Build history of the part. All positions in model axes, mm. A direction names the side the tool comes from. Give positions to 0.01 mm unless a question says otherwise; leave off trailing zeros. Order: outer loops, then holes, each group sorted by start corner. A loop starts at its lowest first (then second) coordinate and runs counter-clockwise, first axis right, second up. Notation, with made-up numbers: (2.25, -16.5) - (27.25, -16.5) arc R17 cw to (27.25, 4.5) - close; hole circle Ø1 at (54, 55). An arc over 180 degrees is marked (long way). Write each question's results on one line, items separated by ' | '. Start each with the question number.
from build123d import *

# Parameters (mm, degrees)
SKETCH1_W             = 80
SKETCH1_H             = 100
BOSS_EXTRUDE1_DEPTH   = 3.5
SKETCH3_W             = 56
SKETCH3_H             = 88
BOSS_EXTRUDE2_DEPTH   = 21.5
SKETCH4_W             = 50
SKETCH4_H             = 82
CUT_EXTRUDE4_DEPTH    = 16
CUT_EXTRUDE5_DEPTH    = 6
SKETCH8_W             = 30
SKETCH8_H             = 5
CUT_EXTRUDE6_DEPTH    = 6
CUT_EXTRUDE7_REACH    = 112.567
SKETCH9_W             = 40
SKETCH9_H             = 12
F_4_0MM_DOWEL_HOLE1_D = 4
FILLET1_R             = 7
FILLET2_R             = 2
FILLET3_R             = 1
FILLET4_R             = 2


# Some blends are built 0.0001 mm under size
with BuildPart() as part:
    # Sketch1 → Boss-Extrude1 (new body)
    with BuildSketch(Plane.XY):
        Rectangle(SKETCH1_W, SKETCH1_H)
    extrude(amount=BOSS_EXTRUDE1_DEPTH)

    # Sketch3 → Boss-Extrude2 (add)
    with BuildSketch(Plane.XY.offset(3.5)):
        Rectangle(SKETCH3_W, SKETCH3_H)
    extrude(amount=BOSS_EXTRUDE2_DEPTH)

    # Sketch4 → Cut-Extrude4 (cut)
    with BuildSketch(Plane(origin=(0, 0, 0), x_dir=(-1, 0, 0), z_dir=(0, 0, -1))):
        Rectangle(SKETCH4_W, SKETCH4_H)
    extrude(amount=-CUT_EXTRUDE4_DEPTH, mode=Mode.SUBTRACT)

    # Sketch7 → Cut-Extrude5 (cut)
    with BuildSketch(Plane(origin=(0, 0, 16), x_dir=(-1, 0, 0), z_dir=(0, 0, -1))):
        Polygon((-18, 41), (18, 41), (18, 34), (25, 34), (25, -34), (18, -34), (18, -41), (-18, -41), (-18, -34), (-25, -34), (-25, 34), (-18, 34), align=None)
    extrude(amount=-CUT_EXTRUDE5_DEPTH, mode=Mode.SUBTRACT)

    # Sketch8 → Cut-Extrude6 (cut)
    with BuildSketch(Plane.XY.offset(25)):
        with Locations((0, -17)):
            Rectangle(SKETCH8_W, SKETCH8_H)
    cut_extrude6 = extrude(amount=-CUT_EXTRUDE6_DEPTH, mode=Mode.SUBTRACT)

    # Mirror1: Cut-Extrude6 across plane
    add(cut_extrude6.mirror(Plane.ZX), mode=Mode.SUBTRACT)

    # Sketch9 → Cut-Extrude7 (cut, up to next)
    with BuildSketch(Plane.XZ.offset(50), mode=Mode.PRIVATE) as cut_extrude7_sk1:
        with Locations((0, 6)):
            Rectangle(SKETCH9_W, SKETCH9_H)
    cut_extrude7_tool1 = extrude(cut_extrude7_sk1.sketch, amount=-CUT_EXTRUDE7_REACH, mode=Mode.PRIVATE) & part.part
    add(cut_extrude7_tool1.solids().sort_by_distance((0, -50, 6))[0], mode=Mode.SUBTRACT)

    # Ø4.0mm Dowel Hole1 (through all)
    with Locations(Plane(origin=(0, 0, 0), x_dir=(-1, 0, 0), z_dir=(0, 0, -1))):
        with Locations((-35, 45), (35, 45), (35, -45), (-35, -45)):
            Hole(F_4_0MM_DOWEL_HOLE1_D / 2)

    # Fillet1
    fillet1_edges = [part.edges().sort_by_distance(p)[0] for p in [
        (-18, 34, 19),
        (18, 34, 19),
        (18, -34, 19),
        (-18, -34, 19),
    ]]
    fillet(fillet1_edges, radius=FILLET1_R - 0.0001)  # a hair under: the kernel refuses the full size

    # Fillet2
    fillet2_edges = [part.edges().sort_by_distance(p)[0] for p in [
        (28, -44, 14.25),
        (28, 44, 14.25),
        (-28, 44, 14.25),
        (-28, -44, 14.25),
        (28, 0, 25),
        (0, 44, 25),
        (-28, 0, 25),
        (15, -14.5, 23.5),
        (15, -19.5, 23.5),
        (-15, -19.5, 23.5),
        (-15, -14.5, 23.5),
        (15, 19.5, 23.5),
        (15, 14.5, 23.5),
        (-15, 14.5, 23.5),
        (-15, 19.5, 23.5),
    ]]
    fillet(fillet2_edges, radius=FILLET2_R)

    # Fillet3
    fillet3_edges = [part.edges().sort_by_distance(p)[0] for p in [
        (-40, 0, 3.5),
        (23, -44, 3.5),
        (30, -50, 3.5),
        (-30, -50, 3.5),
        (28, 0, 3.5),
        (-23, -44, 3.5),
        (-28, 0, 3.5),
        (0, 44, 3.5),
        (27.414213562, -43.414213562, 3.5),
        (-27.414213562, -43.414213562, 3.5),
        (-27.414213562, 43.414213562, 3.5),
        (27.414213562, 43.414213562, 3.5),
        (40, 0, 3.5),
        (0, 50, 3.5),
    ]]
    fillet(fillet3_edges, radius=FILLET3_R)

    # Fillet4
    # the kernel refuses this fillet: 2 mm, written as the material it takes off along each edge
    with BuildSketch(Plane(origin=(-26, -42, 23), x_dir=(0, 0, 1), z_dir=(0, -1, 0))) as fillet4_piece_1_section:
        Polygon((0, 0), (FILLET4_R, 0), (FILLET4_R, FILLET4_R), (0, FILLET4_R), align=None)
    fillet4_piece_1 = extrude(amount=FILLET4_R, mode=Mode.PRIVATE)
    fillet4_piece_1 = fillet4_piece_1 - Plane(origin=(-26, -42, 23), x_dir=(0.7071067811865475, 0, -0.7071067811865475), z_dir=(0, -1, 0)) * Sphere(FILLET4_R, mode=Mode.PRIVATE)
    add(fillet4_piece_1, mode=Mode.SUBTRACT)
    with BuildSketch(Plane(origin=(26, -42, 23), x_dir=(0, 0, 1), z_dir=(0, -1, 0))) as fillet4_piece_2_section:
        Polygon((0, 0), (FILLET4_R, 0), (FILLET4_R, -FILLET4_R), (0, -FILLET4_R), align=None)
    fillet4_piece_2 = extrude(amount=FILLET4_R, mode=Mode.PRIVATE)
    fillet4_piece_2 = fillet4_piece_2 - Plane(origin=(26, -42, 23), x_dir=(-0.7071067811865475, 0, -0.7071067811865475), z_dir=(0, -1, 0)) * Sphere(FILLET4_R, mode=Mode.PRIVATE)
    add(fillet4_piece_2, mode=Mode.SUBTRACT)
    with BuildSketch(Plane(origin=(26, -44, 25), x_dir=(0, 0, -1), z_dir=(-1, 0, 0))) as fillet4_piece_3:
        with BuildLine():
            CenterArc((FILLET4_R, -FILLET4_R), FILLET4_R, 90, 90)
            Line((0, -FILLET4_R), (0, 0))
            Line((0, 0), (FILLET4_R, 0))
        make_face()
    extrude(amount=52, mode=Mode.SUBTRACT)


solid = part.part
Item 1: Cut at D-D, the plane x = 31. List the corners of the cut face in (y, z), then the cut area to 3 significant figures.
Item 2: Flat gauge pins, fed straight in: pin 1 Ø4 at (y, z) = (11.5, 18) entering from +X; pin 2 Ø5 at (y, z) = (3, 8.5) entering from -X; pin 3 Ø0.9 at (x, z) = (2, 23.5) entering from +Y; pin 4 Ø3 at (x, y) = (-35, 45) entering from +Z. Where does each tip first touch, or does it go through?
Item 3: Cut at B-B, the plane y = -21.5. List the corners of the cut face in (x, z).
Item 4: Probe line 1 along Y through (x, z) = (-35, 2.7); line 2 along X through (y, z) = (-4.5, 19.75); line 3 along Y through (x, z) = (9.5, 18.25). List the from-to ranges inside material, lowest first. Write a range as from..to.
Item 5: Cut at A-A, the plane x = -35. List the corners of the cut face in (y, z).
Item 6: Two-plate mould, pull along X, no slides. Class faces 6 (the flat face through (-30, -50, 1)), 7 (the flat face through (40, -1, 1)), 8 (the cylindrical face through (14.4, 15.07, 23.48)): +X half, -X half, draft (parallel to the pull), parting line (faces both ways), or undercut.
Item 7: Which spindle directions (+Z, -Z, +X, -X, +Y, -Y) get a long thin tool onto all of the face, cutting with end or side? Do faces 1 (the flat face through (22, -38, 16)), 2 (the flat face through (0, 44, 14)), 3 (the flat face through (-27, 12, 0)), 4 (the cylindrical face through (14.43, -15.1, 23.48)), 5 (the cylindrical face through (27.4, 0.59, 24.43)). Say none if no direction does.
Values found:
1) outline: (-50, 0) - (50, 0) - (50, 2.5) arc R1 ccw to (49, 3.5) - (-49, 3.5) arc R1 ccw to (-50, 2.5) - close | area: 350 mm2
2) pin 1: stops at x = 28 | pin 2: stops at x = -28 | pin 3: stops at y = 44 | pin 4: passes through
3) outline: (-40, 0) - (-25, 0) - (-25, 22) - (25, 22) - (25, 0) - (40, 0) - (40, 2.5) arc R1 ccw to (39, 3.5) - (29, 3.5) arc R1 cw to (28, 4.5) - (28, 23) arc R2 ccw to (26, 25) - (-26, 25) arc R2 ccw to (-28, 23) - (-28, 4.5) arc R1 cw to (-29, 3.5) - (-39, 3.5) arc R1 ccw to (-40, 2.5) - close
4) line 1: y = -49.98..-47, -43..43, 47..49.98 | line 2: x = -28..-25, 25..28 | line 3: y = -44..-41, 41..44
5) outline: (-50, 0) - (-47, 0) - (-47, 3.5) - (-49, 3.5) arc R1 ccw to (-50, 2.5) - close; (-43, 0) - (43, 0) - (43, 3.5) - (-43, 3.5) - close; (47, 0) - (50, 0) - (50, 2.5) arc R1 ccw to (49, 3.5) - (47, 3.5) - close
6) face 6: draft | face 7: +X half | face 8: undercut
7) face 1: -Z | face 2: +Z, +X, -X, +Y | face 3: -Z, +X, -X, +Y, -Y | face 4: +Z, -Z | face 5: +Z, +X, +Y, -Y
